```python
from build123d import *

# Parameters (mm, degrees)
SKETCH_W        = 25.2
SKETCH_H        = 25.2
PAD_DEPTH       = 13.5
THICKNESS_T     = -3.5
SKETCH001_W     = 18.2
SKETCH001_H     = 10
POCKET_DEPTH    = 3.5
PAD001_DEPTH    = 50
CHAMFER_SIZE    = 1
SKETCH003_W     = 18.2
SKETCH003_H     = 10
POCKET001_DEPTH = 3.5
PAD002_DEPTH    = 50
CHAMFER001_SIZE = 1
FILLET_R        = 2
FILLET001_R     = 2
FILLET002_R     = 2


with BuildPart() as part:
    # Sketch → Pad (new body)
    with BuildSketch(Plane.XY):
        Rectangle(SKETCH_W, SKETCH_H)
    extrude(amount=PAD_DEPTH)

    # Thickness
    thickness_openings = [part.faces().sort_by_distance(p)[0] for p in [
        (0, 0, 13.5),
    ]]
    offset(amount=THICKNESS_T, openings=thickness_openings, kind=Kind.INTERSECTION)

    # Sketch001 (on Face2 of Thickness) → Pocket (cut)
    with BuildSketch(Plane.XZ.offset(12.6)):
        with Locations((0, 8.5)):
            Rectangle(SKETCH001_W, SKETCH001_H)
    extrude(amount=-POCKET_DEPTH, mode=Mode.SUBTRACT)

    # Sketch002 (on Face3 of Pocket) → Pad001 (join)
    with BuildSketch(Plane.XZ.offset(12.6)):
        Polygon((-10.6, 13.5), (-10.6, 2), (10.6, 2), (10.6, 13.5), (9.1, 13.5), (9.1, 3.5), (-9.1, 3.5), (-9.1, 13.5), align=None)
    extrude(amount=PAD001_DEPTH)

    # Chamfer
    chamfer_edges = [part.edges().sort_by_distance(p)[0] for p in [
        (0, -62.6, 2),
        (10.6, -37.6, 2),
        (-10.6, -37.6, 2),
        (10.6, -62.6, 7.75),
        (-10.6, -62.6, 7.75),
    ]]
    chamfer(chamfer_edges, length=CHAMFER_SIZE)

    # Sketch003 (on Face6 of Chamfer) → Pocket001 (cut)
    with BuildSketch(Plane.YZ.offset(12.6)):
        with Locations((0, 8.5)):
            Rectangle(SKETCH003_W, SKETCH003_H)
    extrude(amount=-POCKET001_DEPTH, mode=Mode.SUBTRACT)

    # Sketch004 (on Face6 of Pocket001) → Pad002 (join)
    with BuildSketch(Plane.YZ.offset(12.6)):
        Polygon((10.6, 13.5), (10.6, 2), (-10.6, 2), (-10.6, 13.5), (-9.1, 13.5), (-9.1, 3.5), (9.1, 3.5), (9.1, 13.5), align=None)
    extrude(amount=PAD002_DEPTH)

    # Chamfer001
    chamfer001_edges = [part.edges().sort_by_distance(p)[0] for p in [
        (37.6, -10.6, 2),
        (62.6, -10.6, 7.75),
        (62.6, 0, 2),
        (62.6, 10.6, 7.75),
        (37.6, 10.6, 2),
    ]]
    chamfer(chamfer001_edges, length=CHAMFER001_SIZE)

    # Fillet
    fillet_edges = [part.edges().sort_by_distance(p)[0] for p in [
        (37.6, 9.1, 3.5),
        (10.85, 9.1, 3.5),
        (0, 9.1, 3.5),
        (-9.1, 0, 3.5),
        (-9.1, -10.85, 3.5),
        (-9.1, -37.6, 3.5),
    ]]
    fillet(fillet_edges, radius=FILLET_R)

    # Fillet001
    fillet001_edges = [part.edges().sort_by_distance(p)[0] for p in [
        (9.1, -10.85, 3.5),
    ]]
    fillet(fillet001_edges, radius=FILLET001_R)

    # Fillet002
    fillet002_edges = [part.edges().sort_by_distance(p)[0] for p in [
        (37.6, -9.1, 3.5),
    ]]
    fillet(fillet002_edges, radius=FILLET002_R)


solid = part.part
```
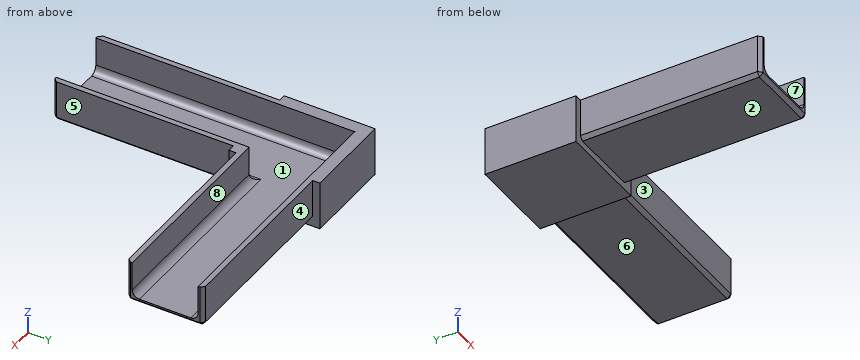
Source: CAD feature listing. Evaluate the final solid. Frame: model axes, mm. Face numbers are marked on the shaded views. A direction names the side the tool comes from. Coordinates: 2 decimals unless noted, no trailing zeros. Loops run counter-clockwise (first coordinate to the right, second up) from the corner with the lowest first, then second, coordinate; pieces in that order, holes last. Notation, with made-up numbers: M 88,-36.75 L 113,-36.75 A26 ccw 113,-17.75 Z; hole C 74,76 d3. An arc over 180 degrees is marked long. Put each result on its own line as item: value. Start each with the question number.
1) Cut plane A-A on z = 9.75. Return the cut outline in (x, y), then the cut area to 3 significant figures.
2) Cut plane D-D on y = -43. Return the cut outline in (x, z), then the cut area to 3 significant figures.
3) Contact query for flat-ended pins moving along their axis: pin 1 Ø2 at (x, y) = (23.5, 2.5) entering from +Z; pin 2 Ø3 at (y, z) = (-42.5, 7.5) entering from -X; pin 3 Ø4 at (y, z) = (6, 8) entering from +X. Output: stop coordinate, or through.
4) Reachability of the marked faces 4, 5, 6, 7 and 8 from +Z, -Z, +X, -X, +Y, -Y: full face, straight path, thin tool, end or side. Return the list, or none.
5) Cut plane C-C on y = -3. Return the cut outline in (x, z), then the cut area to 3 significant figures.
6) Ray query, L1, parallel to Y at x = 23, z = 13; L2, parallel to X at y = -41.5, z = 3.25. Return the intervals inside material, ascending. Write a range as from..to.
7) Pull-direction query (Y, two-part tool) for the marked faces 1, 2 and 3; classes: pulls with the +Y half, pulls with the -Y half, needs draft (parallel to the pull), parting line crosses it, or undercut.
8) Cut plane B-B on x = 0. Return the cut outline in (y, z).
The answers:
1. outline: M -12.6,-12.6 L -10.6,-12.6 L -10.6,-61.6 L -9.6,-62.6 L -9.1,-62.6 L -9.1,9.1 L 62.6,9.1 L 62.6,9.6 L 61.6,10.6 L 12.6,10.6 L 12.6,12.6 L -12.6,12.6 Z; M 9.1,-62.6 L 9.6,-62.6 L 10.6,-61.6 L 10.6,-12.6 L 12.6,-12.6 L 12.6,-10.6 L 61.6,-10.6 L 62.6,-9.6 L 62.6,-9.1 L 9.1,-9.1 Z
1. area: 474 mm²
2. outline: M -10.6,3 L -9.6,2 L 9.6,2 L 10.6,3 L 10.6,13.5 L 9.1,13.5 L 9.1,5.5 A2 cw 7.1,3.5 L -7.1,3.5 A2 cw -9.1,5.5 L -9.1,13.5 L -10.6,13.5 Z
2. area: 62.5 mm²
3. pin 1: stops at z = 3.5
3. pin 2: stops at x = -10.6
3. pin 3: stops at x = -9.1
4. face 4: +Z, -Z, +X, +Y
4. face 5: +Z, -Z, +X, -Y
4. face 6: -Z, +X, +Y, -Y
4. face 7: +Z, -Y
4. face 8: +Z, +X
5. outline: M -12.6,0 L 12.6,0 L 12.6,2 L 61.6,2 L 62.6,3 L 62.6,3.5 L -7.1,3.5 A2 cw -9.1,5.5 L -9.1,13.5 L -12.6,13.5 Z
5. area: 199 mm²
6. L1: y = -10.6..-9.1, 9.1..10.6
6. L2: x = -10.6..10.6
7. face 1: undercut
7. face 2: needs draft
7. face 3: pulls with the -Y half
8. outline: M -62.6,3 L -61.6,2 L -12.6,2 L -12.6,0 L 12.6,0 L 12.6,13.5 L 9.1,13.5 L 9.1,5.5 A2 cw 7.1,3.5 L -62.6,3.5 Z
